CAD build for the part. Positions are in the model's coordinates, mm. A direction names the side the tool comes from. Round coordinates to 2 decimals unless told otherwise and drop trailing zeros. Write each loop counter-clockwise with the first axis right and the second up, starting at its lowest first coordinate (ties: lowest second). Pieces come first, ordered by that corner, then holes. Notation, with made-up numbers: (43, 72) -> (65, 72) arc R30 ccw to (65, 95) -> close; hole circle Ø7 at (76.25, 89.25). An arc over 180 degrees is marked (long way). Put each result on its own line as item: value. Start each with the question number.
1. Drill centre lines: line 1 (X direction, y = 1.4, z = -6.15); line 2 (X direction, y = 2.2, z = -1); line 3 (Z direction, x = -33, y = 1.2). Where is each one in solid material? Low to high. Write a range as from..to.
2. Saw through at C-C on x = 22. List the corners of the cut face in (y, z), and give its area (3 significant figures).
3. Pull direction X, two halves, no side cores. Call faces 1 (the flat face through (-1, 1, -10.15)), 2 (the flat face through (-48.25, 1, 0)), 3 (the flat face through (21.29, 3, 2.44)): pulls with the +X half, pulls with the -X half, needs draft (parallel to the pull), parting line crosses it, or undercut.
4. Saw through at D-D on x = -44. List the corners of the cut face in (y, z), and give its area (3 significant figures).
5. 3-axis set-ups, long thin cutter, end or side, ignore diameter. For faces 4 (the flat face through (-44, 5, 0)), 5 (the cylindrical face through (-20.8, 4, 1.6)): which of +Z, -Z, +X, -X, +Y, -Y reach the whole face in a straight line?
6. Saw through at A-A on z = -6.15. List the corners of the cut face in (x, y).
7. Saw through at B-B on x = 33. List the corners of the cut face in (y, z), and give its area (3 significant figures).
8. Flat gauge pins, fed straight in: P1, Ø0.8, axis at y = 2.5, z = 0.5, coming from the +X side; P2, Ø0.5, axis at y = 2.5, z = 0.5, coming from the -X side; P3, Ø2, axis at x = 28.5, z = -5.5, coming from the +Y side. Where does each tip first touch, or does it go through?
from build123d import *

# Parameters (mm, degrees)
EXTRUDE_2_DEPTH          = 2
CUT_EXTRUDE_3_DEPTH      = 50.346580429
CUT_EXTRUDE_3_DEPTH_BACK = 50.346580429
SKETCH_2_R               = 1.5
SKETCH_3_W               = 6
SKETCH_3_H               = 9
EXTRUDE_3_DEPTH          = 3
EXTRUDE_START            = 3
SKETCH_4_R               = 2
SKETCH_4_R_2             = 2.38964589
EXTRUDE_4_DEPTH          = 2


with BuildPart() as part:
    # 草图1 → 凸台-拉伸2 (new body)
    with BuildSketch(Plane(origin=(0, 0, 0), x_dir=(1, 0, 0), z_dir=(0, 1, 0))):
        with BuildLine():
            Line((46.25, -10.15), (-46.25, -10.15))
            ThreePointArc((-46.25, -10.15), (-47.664213562, -9.564213562), (-48.25, -8.15))
            Line((-48.25, -8.15), (-48.25, 8.15))
            ThreePointArc((-48.25, 8.15), (-47.664213562, 9.564213562), (-46.25, 10.15))
            Line((-46.25, 10.15), (46.25, 10.15))
            ThreePointArc((46.25, 10.15), (47.664213562, 9.564213562), (48.25, 8.15))
            Line((48.25, 8.15), (48.25, -8.15))
            ThreePointArc((48.25, -8.15), (47.664213562, -9.564213562), (46.25, -10.15))
        make_face()
    extrude(amount=EXTRUDE_2_DEPTH)

    # 草图2 → 切除-拉伸3 (cut, two sides: drawn at the far end of the back side and taken through both)
    with BuildSketch(Plane(origin=(0, 0, 0), x_dir=(1, 0, 0), z_dir=(0, 1, 0)).offset(-CUT_EXTRUDE_3_DEPTH_BACK)):
        with Locations(Location((-33, 6.15, 0), (0, 0, 270))):
            Circle(SKETCH_2_R)
        with Locations(Location((33, 6.15, 0), (0, 0, 270))):
            Circle(SKETCH_2_R)
    extrude(amount=CUT_EXTRUDE_3_DEPTH + CUT_EXTRUDE_3_DEPTH_BACK, mode=Mode.SUBTRACT)

    # 草图3 → 凸台-拉伸3 (add)
    with BuildSketch(Plane(origin=(0, 0, 0), x_dir=(1, 0, 0), z_dir=(0, 1, 0))):
        with Locations((-44, -1.5)):
            Rectangle(SKETCH_3_W, SKETCH_3_H)
        with Locations((-22, -1.5)):
            Rectangle(SKETCH_3_W, SKETCH_3_H)
        with Locations((0, -1.5)):
            Rectangle(SKETCH_3_W, SKETCH_3_H)
        with Locations((22, -1.5)):
            Rectangle(SKETCH_3_W, SKETCH_3_H)
        with Locations((44, -1.5)):
            Rectangle(SKETCH_3_W, SKETCH_3_H)
    extrude(amount=EXTRUDE_3_DEPTH)

    # 草图4 → 凸台-拉伸4 (add)
    with BuildSketch(Plane(origin=(0, 0, 0), x_dir=(1, 0, 0), z_dir=(0, 1, 0)).offset(EXTRUDE_START)):
        with Locations(Location((-44, 0, 0), (0, 0, 90))):
            Circle(SKETCH_4_R)
        with Locations(Location((-22, 0, 0), (0, 0, 90))):
            Circle(SKETCH_4_R)
        with Locations(Location((0, 0, 0), (0, 0, 90))):
            Circle(SKETCH_4_R)
        with Locations(Location((22, 0, 0), (0, 0, 90))):
            Circle(SKETCH_4_R_2)
        with Locations(Location((44, 0, 0), (0, 0, 90))):
            Circle(SKETCH_4_R)
    extrude(amount=EXTRUDE_4_DEPTH)


solid = part.part
Return value:
1. line 1: x = -48.25..-34.5, -31.5..31.5, 34.5..48.25
1. line 2: x = -47..-41, -25..-19, -3..3, 19..25, 41..47
1. line 3: z = -10.15..-7.65, -4.65..10.15
2. outline: (0, -10.15) -> (2, -10.15) -> (2, -3) -> (3, -3) -> (3, -2.39) -> (5, -2.39) -> (5, 2.39) -> (3, 2.39) -> (3, 6) -> (2, 6) -> (2, 10.15) -> (0, 10.15) -> close
2. area: 59.2 mm^2
3. face 1: needs draft
3. face 2: pulls with the -X half
3. face 3: undercut
4. outline: (0, -10.15) -> (2, -10.15) -> (2, -3) -> (3, -3) -> (3, -2) -> (5, -2) -> (5, 2) -> (3, 2) -> (3, 6) -> (2, 6) -> (2, 10.15) -> (0, 10.15) -> close
4. area: 57.6 mm^2
5. face 4: +Z, -Z, +X, -X, +Y
5. face 5: +Y
6. outline: (-48.25, 0) -> (-34.5, 0) -> (-34.5, 2) -> (-48.25, 2) -> close; (-31.5, 0) -> (31.5, 0) -> (31.5, 2) -> (-31.5, 2) -> close; (34.5, 0) -> (48.25, 0) -> (48.25, 2) -> (34.5, 2) -> close
7. outline: (0, -10.15) -> (2, -10.15) -> (2, -7.65) -> (0, -7.65) -> close; (0, -4.65) -> (2, -4.65) -> (2, 10.15) -> (0, 10.15) -> close
7. area: 34.6 mm^2
8. P1: stops at x = 47
8. P2: stops at x = -47
8. P3: stops at y = 2
